Autodesk Inventor part; units mm, degrees
ref_plane "YZ Plane" through (0, 0, 0) normal (1, 0, 0) x (0, 1, 0)
ref_plane "XZ Plane" through (0, 0, 0) normal (0, 1, 0) x (-1, 0, 0)
ref_plane "XY Plane" through (0, 0, 0) normal (0, 0, 1) x (1, 0, 0)
sketch "Skizze1" plane through (0, 0, 0) normal (0, 0, 1) x (1, 0, 0)
  line L0 (0, 0) -> (0, -0.02)
  line L1 (0, -0.02) -> (-2.5, -0.02)
  arc A0 (-3.3195, 0.4069) -> (-2.5, -0.02) centre (-2.5, 0.98) ccw
  line L2 (-3.3195, 0.4069) -> (-4.1969, 1.6616)
  arc A1 (-4.1969, 1.6616) -> (-5, 2.08) centre (-5, 1.1) ccw
  line L3 (-5, 2.08) -> (-6.68, 2.08)
  line L4 (-6.68, 2.08) -> (-6.68, 2.1)
  line L5 (-6.68, 2.1) -> (-5, 2.1)
  arc A2 (-4.1805, 1.6731) -> (-5, 2.1) centre (-5, 1.1) ccw
  line L6 (-4.1805, 1.6731) -> (-3.3031, 0.4184)
  line L7 (-2.5, 0) -> (0, 0)
  arc A3 (-3.3031, 0.4184) -> (-2.5, 0) centre (-2.5, 0.98) ccw
  dimension "d0" = 0.02
  dimension "d2" = 10
  dimension "d3" = 0.02
  dimension "d4" = 1
  dimension "d5" = 2.1
  dimension "d6" = 5
revolve "Umdrehung1" add sketch "Skizze1" angle 360 about axis through (0, 0, 0) along (0, -1, 0)
sketch "Skizze2" plane through (0, -0.02, 0) normal (0, -1, 0) x (1, 0, 0)
  line L0 (0, 0) -> (0, 2)
  line L1 (0, 2) -> (0.25, 2)
  line L2 (0.25, 2) -> (0.25, 0.25)
  line L3 (0.25, 0.25) -> (2, 0.25)
  line L4 (2, 0.25) -> (2, 0)
  line L5 (2, 0) -> (0, 0)
  arc A0 (2, 0) -> (1.75, 0.25) centre (1.75, 0) ccw
  arc A1 (0.25, 1.75) -> (0, 2) centre (0, 1.75) ccw
  arc A2 (-1.75, 0.25) -> (-2, 0) centre (-1.75, 0) ccw
  line L6 (-2, 0.25) -> (-0.25, 0.25)
  line L7 (-0.25, 2) -> (0, 2)
  arc A3 (0, 2) -> (-0.25, 1.75) centre (0, 1.75) ccw
  line L8 (-0.25, 0.25) -> (-0.25, 2)
  line L9 (-2, 0) -> (-2, 0.25)
  arc A4 (-0.25, -1.75) -> (0, -2) centre (0, -1.75) ccw
  line L10 (-0.25, -2) -> (-0.25, -0.25)
  line L11 (-2, -0.25) -> (-2, 0)
  arc A5 (-2, 0) -> (-1.75, -0.25) centre (-1.75, 0) ccw
  line L12 (-0.25, -0.25) -> (-2, -0.25)
  line L13 (0, -2) -> (-0.25, -2)
  arc A6 (1.75, -0.25) -> (2, 0) centre (1.75, 0) ccw
  line L14 (2, -0.25) -> (0.25, -0.25)
  line L15 (0.25, -2) -> (0, -2)
  arc A7 (0, -2) -> (0.25, -1.75) centre (0, -1.75) ccw
  line L16 (0.25, -0.25) -> (0.25, -2)
  line L17 (2, 0) -> (2, -0.25)
  point P0 (0, 2)
  point P1 (-2, 0)
  point P2 (0, -2)
  dimension "d8" = 4
  dimension "d9" = 0.5
  dimension "d12" = 360
extrude "Extrusion1" cut sketch "Skizze2" against normal through all contours L5 A6 L14 L16 A7 A4 L10 L12 A5 A2 L6 L8 A3 L0 | L0 A1 L2 L3 A0 L5
equation "\"d3\" = d0"
equation "\"Biegeradius\" = Stärke"
equation "\"BreiteBiegungsfreistellung\" = Stärke"
equation "\"TiefeBiegungsfreistellung\" = 0.5 * Stärke"
equation "\"GrößeEckenfreistellung\" = 4 * Stärke"
equation "\"MinimalRest\" = 2 * Stärke"
equation "\"Übergangsradius\" = Biegeradius"
equation "\"JacobiRadiusGröße\" = Biegeradius"
equation "\"Abstandsgröße\" = Stärke"
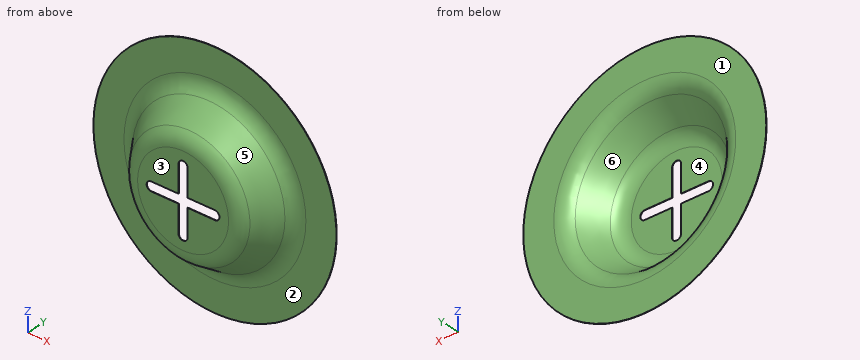
Model file for the job. Use its own axes, mm. Face numbers are marked on the shaded views. A direction names the side the tool comes from. Coordinates: 2 decimals unless noted, no trailing zeros. Loops run counter-clockwise (first coordinate to the right, second up) from the corner with the lowest first, then second, coordinate; pieces in that order, holes last. Notation, with made-up numbers: (-12, 30.25) - (37, 30.25) arc R19 cw to (37, 63.25) - close; hole circle Ø7 at (1.25, 85). An arc over 180 degrees is marked (long way). Write item = value, one per line. Start each with the question number.
Item 1: 3-axis set-ups, long thin cutter, end or side, ignore diameter. For the marked faces 1 and 2: which of +Z, -Z, +X, -X, +Y, -Y reach the whole face in a straight line?
Item 2: Saw through at C-C, the plane y = 0.85. List the corners of the cut face in (x, z).
Item 3: Drop flat-ended pins along their axis: pin 1 Ø4 at (x, z) = (2.5, -4.5) entering from -Y; pin 2 Ø2.5 at (x, z) = (-0.5, -0.5) entering from +Y; pin 3 Ø1.5 at (x, z) = (-3, 2.5) entering from +Y. Give the stop position or say it passes through.
Item 4: Pull direction Z, two halves, no side cores. Call the marked faces 3, 4, 5 and 6: +Z half, -Z half, draft (parallel to the pull), parting line (faces both ways), or undercut.
Answers:
q1.face_1 = +Z, -Z, +X, -X, +Y
q1.face_2 = -Y
q2.outline = circle Ø7.26 at (0, 0); hole circle Ø7.21 at (0, 0)
q3.pin_1 = 0.22
q3.pin_2 = 0
q3.pin_3 = 2.04
q4.face_3 = draft
q4.face_4 = undercut
q4.face_5 = parting line
q4.face_6 = undercut
